Input: part model. Units: mm. Frame: model coordinates. A direction names the side the tool comes from. Give positions to 0.01 mm unless a question says otherwise; leave off trailing zeros. Loops run counter-clockwise (first coordinate to the right, second up) from the corner with the lowest first, then second, coordinate; pieces in that order, holes last.
from build123d import *

# Parameters (mm, degrees)
BOSS_EXTRUDE1_DEPTH = 12.7
SKETCH2_R           = 1.4351
BOSS_EXTRUDE2_DEPTH = 3.81
CUT_EXTRUDE1_DEPTH  = 34.12884745
FILLET1_R           = 0.254


with BuildPart() as part:
    # Sketch1 → Boss-Extrude1 (new body)
    with BuildSketch(Plane(origin=(0, 0, 0), x_dir=(0, 0, -1), z_dir=(1, 0, 0))):
        with BuildLine():
            ThreePointArc((-23.9, 1.3716), (-17.832549445, 0.343974693), (-11.688312193, 0))
            Line((-11.688312193, 0), (0, 0))
            Line((0, 0), (0, 9.652))
            Line((0, 9.652), (-3.175, 9.652))
            Line((-3.175, 9.652), (-3.175, 3.302))
            Line((-3.175, 3.302), (-29.035657895, 3.302))
            Line((-29.035657895, 3.302), (-29.035657895, 2.54))
            Line((-29.035657895, 2.54), (-23.9, 1.3716))
        make_face()
    extrude(amount=BOSS_EXTRUDE1_DEPTH)

    # Sketch2 → Boss-Extrude2 (add)
    with BuildSketch(Plane(origin=(0, 3.302, 0), x_dir=(1, 0, 0), z_dir=(0, 1, 0))):
        with Locations(Location((6.35, -25.4, 0), (0, 0, 90))):
            Circle(SKETCH2_R)
    extrude(amount=BOSS_EXTRUDE2_DEPTH)

    # Sketch3 → Cut-Extrude1 (cut, through all)
    with BuildSketch(Plane(origin=(12.7, 0, 0), x_dir=(0, 0, -1), z_dir=(1, 0, 0))):
        Polygon((-26.8351, 3.556), (-23.9649, 5.207), (-23.9649, 7.112), (-26.8351, 7.112), align=None)
    extrude(amount=-CUT_EXTRUDE1_DEPTH, mode=Mode.SUBTRACT)

    # Fillet1
    fillet1_edges = [part.edges().sort_by_distance(p)[0] for p in [
        (7.7851, 4.3815, 25.4),
    ]]
    fillet(fillet1_edges, radius=FILLET1_R)


solid = part.part
(1) Reachability of faces 1 (the cylindrical face through (6.9, 3.862, 24.074)), 2 (the flat face through (6, 0, 6)) from +Z, -Z, +X, -X, +Y, -Y: full face, straight path, thin tool, end or side. Return the list, or none.
Values follow:
face 1: +Y
face 2: +Z, -Z, +X, -X, -Y
(2) Cut plane B-B (z = 9). Return the cut outline in (x, y).
Values follow:
outline: (0, 0) - (12.7, 0) - (12.7, 3.3) - (0, 3.3) - close
(3) Ray query, probe 1 along Y at (x, z) = (4.25, 9.5); probe 2 along Z at (x, y) = (11.5, 5.5) (3 decimals); probe 3 along Z at (x, y) = (7, 4) (3 decimals). Return the intervals inside material, ascending.
Values follow:
probe 1: y = 0 to 3.3
probe 2: z = 0 to 3.175
probe 3: z = 0 to 3.175, 24.121 to 26.063
(4) Cut plane A-A (x = 1.5). Return the cut outline in (y, z) (3 decimals), and give its area (3 significant figures).
Values follow:
outline: (0, 0) - (9.652, 0) - (9.652, 3.175) - (3.302, 3.175) - (3.302, 29.036) - (2.54, 29.036) - (1.372, 23.9) arc R55.048 ccw to (0, 11.688) - close
area: 100 mm2
(5) Cut plane C-C (y = 6.5). Return the cut outline in (x, z) (3 decimals).
Values follow:
outline: (0, 0) - (12.7, 0) - (12.7, 3.175) - (0, 3.175) - close
(6) Mould query, pull axis Z, two halves, no side actions, for faces 3 (the flat face through (6.37, 4.3, 25.54)), 4 (the flat face through (0, 3, 10)), 5 (the flat face through (6, 5, 0)), 6 (the flat face through (6, 3.302, 16)). Classes: +Z half, -Z half, draft (parallel to the pull), parting line (faces both ways), or undercut.
Values follow:
face 3: +Z half
face 4: draft
face 5: -Z half
face 6: undercut
(7) Pin query (flat end, axial travel): pin 1 Ø6.5 at (x, z) = (7.5, 18) entering from +Y. Return the tip coordinate at first contact, or that it passes through.
Values follow:
pin 1: stops at y = 3.3
